from build123d import *

# Parameters (mm, degrees)
F0_W     = 105
F0_H     = 60
F0_W_2   = 72
F0_H_2   = 25
F1_DEPTH = 2
F2_W     = 105
F2_H     = 60
F2_W_2   = 101
F2_H_2   = 56
F3_DEPTH = 16.5
F4_W     = 2
F4_H     = 9
F4_H_2   = 13
F5_DEPTH = 9
F6_R     = 2
F7_R     = 2
F8_W     = 2
F8_H     = 13
F9_DEPTH = 4


with BuildPart() as f1:
    # F0 (on Top) → F1 (new body)
    with BuildSketch(Plane.XY):
        Rectangle(F0_W, F0_H)
        with Locations((6, 5)):
            Rectangle(F0_W_2, F0_H_2, mode=Mode.SUBTRACT)
    extrude(amount=F1_DEPTH)

    # F2 (on face) → F3 (join)
    with BuildSketch(Plane.XY.offset(2)):
        Rectangle(F2_W, F2_H)
        Rectangle(F2_W_2, F2_H_2, mode=Mode.SUBTRACT)
    extrude(amount=F3_DEPTH)

    # F4 (on face) → F5 (cut)
    with BuildSketch(Plane.XY.offset(18.5)):
        with Locations((-51.5, 8)):
            Rectangle(F4_W, F4_H)
        with Locations((-51.5, -12.5)):
            Rectangle(F4_W, F4_H_2)
    extrude(amount=-F5_DEPTH, mode=Mode.SUBTRACT)

    # F6
    f6_edges = [f1.edges().sort_by_distance(p)[0] for p in [
        (52.5, -30, 9.25),
        (52.5, 30, 9.25),
        (-52.5, -30, 9.25),
        (-52.5, 30, 9.25),
    ]]
    fillet(f6_edges, radius=F6_R)

    # F7
    f7_edges = [f1.edges().sort_by_distance(p)[0] for p in [
        (52.5, 0, 0),
        (0, -30, 0),
        (0, 30, 0),
        (-52.5, 0, 0),
    ]]
    fillet(f7_edges, radius=F7_R)

    # F8 (on face) → F9 (join)
    with BuildSketch(Plane.XY.offset(9.5)):
        with Locations((-51.5, -12.5)):
            Rectangle(F8_W, F8_H)
    extrude(amount=F9_DEPTH)


solid = f1.part
Build history of the part. All positions in model axes, mm. A direction names the side the tool comes from. Round coordinates to 2 decimals unless told otherwise and drop trailing zeros. Write each loop counter-clockwise with the first axis right and the second up, starting at its lowest first coordinate (ties: lowest second). Pieces come first, ordered by that corner, then holes. Notation, with made-up numbers: M 86.5,-37 L 119.5,-37 A32 cw 119.5,-3 Z; hole C 52,16 d1. An arc over 180 degrees is marked long. Answer as a JSON object with one key per item and string values. Group by question number.
(1) Cut at D-D (y = 26). Give the cut face in (x, z), and give its area (3 significant figures).
(2) Drill centre lines: L1, parallel to Y at x = 38.5, z = 11.75; L2, parallel to X at y = 21, z = 4.25; L3, parallel to Z at x = 46, y = 18. Where is each one in solid material? Low to high.
(3) Cut at C-C (x = -23). Give the cut face in (y, z), and give its area (3 significant figures).
(4) Cut at A-A (y = 7.5). Give the cut face in (x, z).
(5) Flat gauge pins, fed straight in: pin 1 (1 mm diameter, centred on x = -51.5, z = 15, fed in from -Y); pin 2 (1.6 mm diameter, centred on y = 4, z = 0.5, fed in from -X); pin 3 (2 mm diameter, centred on x = -52, y = 8, fed in from +Z). Where does each tip first touch, or does it go through?
(6) Mould opens along X. For faces 1 (the cylindrical face through (51.9, -29.43, 10.37)), 2 (the flat face through (-50.5, 0, 8)), 3 (the cylindrical face through (-51.9, -0.39, 0.57)) say: pulls with the +X half, pulls with the -X half, needs draft (parallel to the pull), parting line crosses it, or undercut.
(7) Which spindle directions (+Z, -Z, +X, -X, +Y, -Y) get a long thin tool onto all of the face, cutting with end or side? Do faces 4 (the flat face through (-52, -19, 16)), 5 (the flat face through (-1, 28, 10)), 6 (the flat face through (5, 17.5, 1)), 7 (the cylindrical face through (-51.93, -29.4, 10.37)), 8 (the flat face through (-52.5, 0, 8)). Say none if no direction does.
(8) Cut at B-B (z = 15.75). Give the cut face in (x, y).
Responses:
{
 "1": {"outline": "M -52.5,2 A2 ccw -50.5,0 L 50.5,0 A2 ccw 52.5,2 L 52.5,18.5 L 50.5,18.5 L 50.5,2 L -50.5,2 L -50.5,18.5 L -52.5,18.5 Z", "area": "274 mm2"},
 "2": {"L1": "y = -30 to -28, 28 to 30", "L2": "x = -52.5 to -50.5, 50.5 to 52.5", "L3": "z = 0 to 2"},
 "3": {"outline": "M -30,2 A2 ccw -28,0 L -7.5,0 L -7.5,2 L -28,2 L -28,18.5 L -30,18.5 Z; M 17.5,0 L 28,0 A2 ccw 30,2 L 30,18.5 L 28,18.5 L 28,2 L 17.5,2 Z", "area": "134 mm2"},
 "4": {"outline": "M -52.5,2 A2 ccw -50.5,0 L -30,0 L -30,2 L -50.5,2 L -50.5,9.5 L -52.5,9.5 Z; M 42,0 L 50.5,0 A2 ccw 52.5,2 L 52.5,18.5 L 50.5,18.5 L 50.5,2 L 42,2 Z"},
 "5": {"pin 1": "stops at y = -29.94", "pin 2": "stops at x = -52.37", "pin 3": "stops at z = 9.5"},
 "6": {"face 1": "pulls with the +X half", "face 2": "undercut", "face 3": "pulls with the -X half"},
 "7": {"face 4": "+Z, -X", "face 5": "+Z", "face 6": "+Z, -Z", "face 7": "+Z, -Z, -X, -Y", "face 8": "+Z, -Z, -X, +Y, -Y"},
 "8": {"outline": "M -52.5,-28 A2 ccw -50.5,-30 L 50.5,-30 A2 ccw 52.5,-28 L 52.5,28 A2 ccw 50.5,30 L -50.5,30 A2 ccw -52.5,28 L -52.5,12.5 L -50.5,12.5 L -50.5,28 L 50.5,28 L 50.5,-28 L -50.5,-28 L -50.5,-19 L -52.5,-19 Z; M -52.5,-6 L -50.5,-6 L -50.5,3.5 L -52.5,3.5 Z"}
}
